Geometry: final body of the model. Coordinates: model frame, mm. Face numbers are marked on the shaded views. A direction names the side the tool comes from. Coordinates: 2 decimals unless noted, no trailing zeros. Write each loop counter-clockwise with the first axis right and the second up, starting at its lowest first coordinate (ties: lowest second). Pieces come first, ordered by that corner, then holes. Notation, with made-up numbers: M -33.75,-38.75 L 12.25,-38.75 A15 cw 12.25,-26.75 Z; hole C 65.25,-29.5 d5. An arc over 180 degrees is marked long. Write item = value, one per line. Start each with the question number.
Item 1: Reachability of the marked faces 4, 5 and 6 from +Z, -Z, +X, -X, +Y, -Y: full face, straight path, thin tool, end or side. Return the list, or none.
Item 2: Ray query, L1, parallel to Y at x = 10, z = -2.6; L2, parallel to X at y = 7, z = 2; L3, parallel to X at y = 10.5, z = -1.25. Return the intervals inside material, ascending. Write a range as [from, to].
Item 3: Pull-direction query (Y, two-part tool) for the marked faces 1, 2 and 3; classes: +Y half, -Y half, draft (parallel to the pull), parting line (faces both ways), or undercut.
Item 4: Section B-B on y = 12. Output: boundary loops of the cut face in (x, z), plus the area to 3 significant figures.
Item 5: First-contact query: pin 1 Ø4.5 at (y, z) = (10.5, 2) entering from +X; pin 2 Ø4.5 at (x, y) = (11.5, 14) entering from +Z; pin 3 Ø6 at (x, z) = (9.5, 1.5) entering from +Y. Flat tips, straight axial feed; report the tip coordinate or a pass-through.
Item 6: Section A-A on x = 10. Give the number of separate pieces and of enclosed holes in the cut face, plus the area to 3 significant figures.
Item 7: Section D-D on x = 24. Output: boundary loops of the cut face in (y, z).
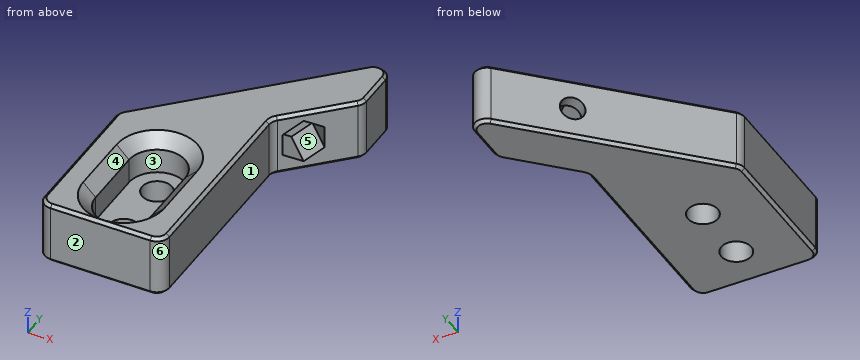
Autodesk Inventor part; units mm, degrees
ref_plane "YZ Plane" through (0, 0, 0) normal (1, 0, 0) x (0, 1, 0)
ref_plane "XZ Plane" through (0, 0, 0) normal (0, 1, 0) x (-1, 0, 0)
ref_plane "XY Plane" through (0, 0, 0) normal (0, 0, 1) x (1, 0, 0)
sketch "Sketch1" plane through (0, 0, 0) normal (0, 0, 1) x (1, 0, 0)
  line L0 (0, 0) -> (20, 0)
  line L1 (20, 0) -> (20, 24)
  line L2 (20, 24) -> (0, 24)
  line L3 (0, 24) -> (0, 0)
  line L4 (0, 24) -> (28.2843, 52.2843)
  line L5 (29.598, 42.2843) -> (29.598, 52.2843)
  line L6 (20, 24) -> (20, 32.6863)
  line L7 (20, 32.6863) -> (29.598, 42.2843)
  line L8 (10, 0) -> (10, 46.8926) construction
  circle A0 centre (10, 17) radius 2.4
  circle A1 centre (10, 7) radius 2.4
  line L9 (28.2843, 52.2843) -> (29.598, 52.2843)
  dimension "d0" = 24
  dimension "d1" = 20
  dimension "d3" = 8
  dimension "d4" = 45
  dimension "d6" = 4.8
  dimension "d7" = 4.8
  dimension "d8" = 7
  dimension "d9" = 7
  dimension "d10" = 10
  dimension "d12" = 40
extrude "Extrusion1" add sketch "Sketch1" along normal mid plane 10
sketch "Sketch2" plane through (0, 0, 5) normal (0, 0, 1) x (1, 0, 0)
  circle A0 centre (10, 17) radius 2.4
  circle A1 centre (10, 7) radius 2.4
  arc A2 (14.5, 17) -> (5.5, 17) centre (10, 17) ccw
  arc A3 (5.5, 7) -> (14.5, 7) centre (10, 7) ccw
  line L0 (5.5, 17) -> (5.5, 7)
  line L1 (14.5, 17) -> (14.5, 7)
  point P0 (0, 0)
  dimension "d15" = 9
  dimension "d16" = 9
extrude "Extrusion2" cut sketch "Sketch2" against normal blind 6
sketch "Sketch4" plane through (0, 24, -5) normal (-0.7071, 0.7071, 0) x (-0.7071, -0.7071, 0)
  line L0 (38.7328, 5) -> (-54.2059, 5)
  circle A0 centre (-25, 5) radius 1.9
  line L1 (0, 0) -> (0, 10)
  point P0 (16.9706, 5)
  dimension "d19" = 3.8
  dimension "d20" = 25
extrude "Extrusion3" cut sketch "Sketch4" against normal through all
sketch "Sketch5" plane through (29.598, 42.2843, 5) normal (0.7071, -0.7071, 0) x (-0.7071, -0.7071, 0)
  circle A0 centre (8.8579, 5) radius 1.9
  line L0 (8.8579, 8.5796) -> (11.9579, 6.7898)
  line L1 (11.9579, 6.7898) -> (11.9579, 3.2102)
  line L2 (11.9579, 3.2102) -> (8.8579, 1.4204)
  line L3 (8.8579, 1.4204) -> (5.7579, 3.2102)
  line L4 (5.7579, 3.2102) -> (5.7579, 6.7898)
  line L5 (5.7579, 6.7898) -> (8.8579, 8.5796)
  point P0 (50.8284, 5)
  dimension "d23" = 6.2
extrude "Extrusion4" cut sketch "Sketch5" against normal blind 6
fillet "Fillet1" radius 2 7 edges at (0, 0, 0) (20, 0, 0) (0, 24, 0) (20, 32.6863, 0) (29.598, 42.2843, 0) (29.598, 52.2843, 0) (28.2843, 52.2843, 0)
chamfer "Chamfer1" distance 2 angle 45 4 edges at (5.5, 12, 5) (10, 21.5, 5) (14.5, 12, 5) (10, 2.5, 5)
chamfer "Chamfer2" distance 0.5 angle 45 22 edges at (13.3856, 37.3856, -5) (29.598, 45.9423, -5) (29.4457, 42.3473, -5) (24.799, 37.4853, -5) (20.1522, 32.6232, -5) (20, 16.9289, -5) (19.4142, 0.5858, -5) (10, 0, -5) (0.5858, 0.5858, -5) (0, 12.5858, -5) (0.1522, 23.9369, -5) (13.3856, 37.3856, 5) (0.1522, 23.9369, 5) (0, 12.5858, 5) (0.5858, 0.5858, 5) (10, 0, 5) (19.4142, 0.5858, 5) (20, 16.9289, 5) (20.1522, 32.6232, 5) (24.799, 37.4853, 5) (29.4457, 42.3473, 5) (29.598, 45.9423, 5)
equation "\"d7\" = d6"
equation "\"d9\" = d8"
equation "\"d16\" = d15"
properties part number "_3DPrint"
Responses:
q1.face_4 = +Z
q1.face_5 = none
q1.face_6 = +Z, -Z, +X, -Y
q2.L1 = [0, 4.6], [9.4, 14.6], [19.4, 34]
q2.L2 = [0, 5.5], [14.5, 20]
q2.L3 = [0, 20]
q3.face_1 = draft
q3.face_2 = -Y half
q3.face_3 = undercut
q4.outline = M 0,-4.5 L 0.5,-5 L 19.5,-5 L 20,-4.5 L 20,4.5 L 19.5,5 L 16.5,5 L 14.5,3 L 14.5,-1 L 5.5,-1 L 5.5,3 L 3.5,5 L 0.5,5 L 0,4.5 Z
q4.area = 142 mm²
q5.pin_1 = 20
q5.pin_2 = -1
q5.pin_3 = 36.5
q6.separate_pieces = 3
q6.enclosed_holes = 0
q6.area = 183 mm²
q7.outline = M 36.69,-4.5 L 37.39,-5 L 47.29,-5 L 48,-4.5 L 48,4.5 L 47.29,5 L 37.39,5 L 36.69,4.5 L 36.69,3.04 L 39.74,1.79 L 39.74,-1.79 L 36.69,-3.04 Z
